Work out the finished part from the listing and answer in its coordinate system (mm). Face numbers are marked on the shaded views. A direction names the side the tool comes from. Coordinates: 2 decimals unless noted, no trailing zeros. Loops run counter-clockwise (first coordinate to the right, second up) from the corner with the lowest first, then second, coordinate; pieces in that order, holes last. Notation, with made-up numbers: (29.5, -33) -> (66.5, -33) arc R22 cw to (66.5, -10) -> close; hole circle Ø7 at (56, 51.5). An arc over 180 degrees is marked (long way). Answer as CSV lines item,"result".
```python
from build123d import *

# Parameters (mm, degrees)
SKETCH2_W               = 60
SKETCH2_H               = 60
BOSS_EXTRUDE1_DEPTH     = 170
SKETCH3_W               = 15
SKETCH3_H               = 60
BOSS_EXTRUDE2_DEPTH     = 30
BOSS_EXTRUDE3_DEPTH     = 15
BOSS_EXTRUDE4_START     = -15
BOSS_EXTRUDE4_DEPTH     = 15
SKETCH6_W               = 60
SKETCH6_H               = 27
BOSS_EXTRUDE5_DEPTH     = 30
BOSS_EXTRUDE6_DEPTH     = 27
CUT_EXTRUDE2_DEPTH      = 5
CUT_EXTRUDE2_DEPTH_BACK = 130
CUT_EXTRUDE2_START      = -10
SKETCH8_W               = 50.5
SKETCH8_H               = 50.5
SKETCH9_R               = 11.35
CUT_EXTRUDE3_DEPTH      = 130
SKETCH11_R              = 3.95
CUT_EXTRUDE4_DEPTH      = 232.543759953
SKETCH12_R              = 3.95
CUT_EXTRUDE5_DEPTH      = 232.543759953
CUT_EXTRUDE7_DEPTH      = 30
FILLET2_R               = 5
FILLET3_R               = 5
SKETCH16_W              = 16
SKETCH16_H              = 11.5
CUT_EXTRUDE8_DEPTH      = 71


with BuildPart() as part:
    # Sketch2 → Boss-Extrude1 (new body)
    with BuildSketch(Plane.XY):
        Rectangle(SKETCH2_W, SKETCH2_H)
    extrude(amount=BOSS_EXTRUDE1_DEPTH)

    # Sketch3 → Boss-Extrude2 (add)
    with BuildSketch(Plane(origin=(0, 0, 0), x_dir=(-1, 0, 0), z_dir=(0, 0, -1))):
        with Locations((22.5, 0)):
            Rectangle(SKETCH3_W, SKETCH3_H)
        with Locations((-22.5, 0)):
            Rectangle(SKETCH3_W, SKETCH3_H)
    extrude(amount=BOSS_EXTRUDE2_DEPTH)

    # Sketch4 → Boss-Extrude3 (add)
    with BuildSketch(Plane(origin=(30, 0, 0), x_dir=(0, 0, -1), z_dir=(1, 0, 0))):
        with BuildLine():
            Line((30, 30), (30, -30))
            ThreePointArc((30, -30), (55.138874415, 0), (30, 30))
        make_face()
    extrude(amount=-BOSS_EXTRUDE3_DEPTH)

    # Sketch5 → Boss-Extrude4 (add)
    with BuildSketch(Plane.ZY.offset(30).offset(BOSS_EXTRUDE4_START)):
        with BuildLine():
            Line((-30, -30), (-30, 30))
            ThreePointArc((-30, 30), (-55.138874415, 0), (-30, -30))
        make_face()
    extrude(amount=BOSS_EXTRUDE4_DEPTH)

    # Sketch6 → Boss-Extrude5 (add)
    with BuildSketch(Plane.XY.offset(170)):
        Rectangle(SKETCH6_W, SKETCH6_H)
    extrude(amount=BOSS_EXTRUDE5_DEPTH)

    # Sketch7 → Boss-Extrude6 (add)
    with BuildSketch(Plane(origin=(0, 13.5, 0), x_dir=(1, 0, 0), z_dir=(0, 1, 0))):
        with BuildLine():
            Line((30, -200), (-30, -200))
            ThreePointArc((-30, -200), (0, -225.138874415), (30, -200))
        make_face()
    extrude(amount=-BOSS_EXTRUDE6_DEPTH)

    # Sketch8 → Cut-Extrude2 (cut, two sides: drawn at the far end of the back side and taken through both)
    with BuildSketch(Plane.XY.offset(170).offset(CUT_EXTRUDE2_START - CUT_EXTRUDE2_DEPTH_BACK)):
        Rectangle(SKETCH8_W, SKETCH8_H)
    extrude(amount=CUT_EXTRUDE2_DEPTH + CUT_EXTRUDE2_DEPTH_BACK, mode=Mode.SUBTRACT)

    # Sketch9 → Cut-Extrude3 (cut)
    with BuildSketch(Plane(origin=(0, -13.5, 0), x_dir=(-1, 0, 0), z_dir=(0, -1, 0))):
        with Locations(Location((0, -200, 0), (0, 0, 90))):
            Circle(SKETCH9_R)
    extrude(amount=-CUT_EXTRUDE3_DEPTH, mode=Mode.SUBTRACT)

    # Sketch11 → Cut-Extrude4 (cut, through all)
    with BuildSketch(Plane.ZY.offset(-15)):
        with Locations(Location((-30, 0, 0), (0, 0, 270))):
            Circle(SKETCH11_R)
    extrude(amount=-CUT_EXTRUDE4_DEPTH, mode=Mode.SUBTRACT)

    # Sketch12 → Cut-Extrude5 (cut, through all)
    with BuildSketch(Plane(origin=(-15, 0, 0), x_dir=(0, 0, -1), z_dir=(1, 0, 0))):
        with Locations(Location((30, 0, 0), (0, 0, 270))):
            Circle(SKETCH12_R)
    extrude(amount=-CUT_EXTRUDE5_DEPTH, mode=Mode.SUBTRACT)

    # Sketch14 → Cut-Extrude7 (cut)
    with BuildSketch(Plane(origin=(-15, 0, 0), x_dir=(0, 0, -1), z_dir=(1, 0, 0))):
        Polygon((0, -30), (0, 0), (-33.188384016, -30), align=None)
        Polygon((-33.188384016, 30), (0, 0), (0, 30), align=None)
    extrude(amount=CUT_EXTRUDE7_DEPTH, mode=Mode.SUBTRACT)

    # Fillet2
    fillet2_edges = [part.edges().sort_by_distance(p)[0] for p in [
        (0, 0, 0),
    ]]
    fillet(fillet2_edges, radius=FILLET2_R)

    # Fillet3
    fillet3_edges = [part.edges().sort_by_distance(p)[0] for p in [
        (0, 13.5, 170),
        (0, -13.5, 170),
    ]]
    fillet(fillet3_edges, radius=FILLET3_R)

    # Sketch16 → Cut-Extrude8 (cut)
    with BuildSketch(Plane(origin=(0, 30, 0), x_dir=(1, 0, 0), z_dir=(0, 1, 0))):
        Polygon((16, -151.43), (16, -101.43), (-16, -101.43), (-16, -139.93), (0, -139.93), (0, -151.43), align=None)
        with Locations((-8, -145.68)):
            Rectangle(SKETCH16_W, SKETCH16_H)
    extrude(amount=-CUT_EXTRUDE8_DEPTH, mode=Mode.SUBTRACT)


solid = part.part
```
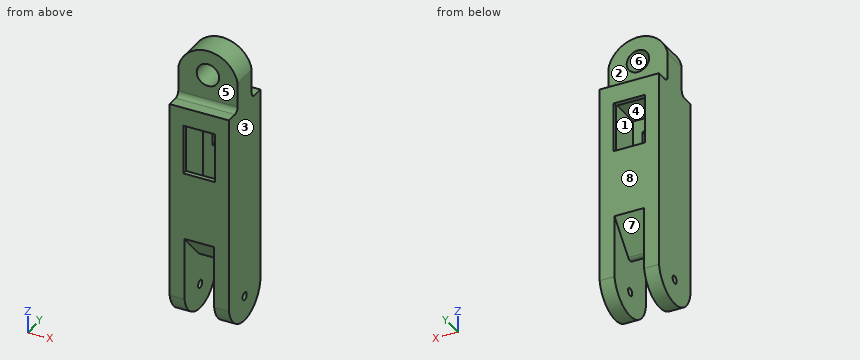
(1) For a pull along X with two mould halves and no side action, classify the marked faces 1, 2 and 3 as pulls with the +X half, pulls with the -X half, needs draft (parallel to the pull), parting line crosses it, or undercut.
Computed values:
face 1,"undercut"
face 2,"needs draft"
face 3,"pulls with the +X half"
(2) A cutting plane is placed at C-C, the plane x = 0. Write down the section's boundary in (y, z).
Computed values:
outline,"(-30, 33.19) -> (-3.71, 4.1) arc R5 ccw to (3.71, 4.1) -> (30, 33.19) -> (30, 101.43) -> (25.25, 101.43) -> (25.25, 30) -> (-25.25, 30) -> (-25.25, 101.43) -> (-30, 101.43) -> close; (-30, 151.43) -> (-25.25, 151.43) -> (-25.25, 165) -> (25.25, 165) -> (25.25, 151.43) -> (30, 151.43) -> (30, 170) -> (18.5, 170) arc R5 cw to (13.5, 175) -> (13.5, 188.65) -> (-13.5, 188.65) -> (-13.5, 175) arc R5 cw to (-18.5, 170) -> (-30, 170) -> close; (-13.5, 211.35) -> (13.5, 211.35) -> (13.5, 225.14) -> (-13.5, 225.14) -> close"
(3) A cutting plane is placed at D-D, the plane y = 21.5. Write down the section's boundary in (x, z) (3 decimals), and give its area (3 significant figures).
Computed values:
outline,"(-30, -46.26) -> (-15, -46.26) -> (-15, 23.785) -> (15, 23.785) -> (15, -46.26) -> (30, -46.26) -> (30, 170) -> (-30, 170) -> close; hole (-25.25, 30) -> (25.25, 30) -> (25.25, 165) -> (-25.25, 165) -> close"
area,"4,060 mm2"
(4) Consider line 1 along X through (y, z) = (7, 200); line 2 along X through (y, z) = (18.5, 131); line 3 along Z through (x, y) = (-20, 0). Determine where each line is inside the solid, lowest interval first.
Computed values:
line 1,"-30 to -11.35, 11.35 to 30"
line 2,"-30 to -25.25, 25.25 to 30"
line 3,"-55.14 to -33.95, -26.05 to 30, 165 to 217.66"
(5) Which of the six approach directions +Z, -Z, +X, -X, +Y, -Y give full straight-line access (tool end or side, diameter ignored) to the marked faces 4, 5, 6, 7 and 8?
Computed values:
face 4,"none"
face 5,"+Z, +X, -X, -Y"
face 6,"+Y, -Y"
face 7,"-Z, +Y"
face 8,"+Z, -Z, +X, -X, +Y"
(6) A cutting plane is placed at A-A, the plane y = 0. Write down the section's boundary in (x, z).
Computed values:
outline,"(-30, -55.14) -> (-15, -55.14) -> (-15, -33.95) -> (-30, -33.95) -> close; (-30, -26.05) -> (-15, -26.05) -> (-15, 2.46) -> (15, 2.46) -> (15, -26.05) -> (30, -26.05) -> (30, 200) arc R30.47 ccw to (-30, 200) -> close; (15, -55.14) -> (30, -55.14) -> (30, -33.95) -> (15, -33.95) -> close; hole (-25.25, 30) -> (25.25, 30) -> (25.25, 165) -> (-25.25, 165) -> close; hole circle Ø22.7 at (0, 200)"
(7) A cutting plane is placed at B-B, the plane z = 137. Write down the section's boundary in (x, y).
Computed values:
outline,"(-30, -30) -> (-16, -30) -> (-16, -25.25) -> (-25.25, -25.25) -> (-25.25, 25.25) -> (-16, 25.25) -> (-16, 30) -> (-30, 30) -> close; (16, -30) -> (30, -30) -> (30, 30) -> (16, 30) -> (16, 25.25) -> (25.25, 25.25) -> (25.25, -25.25) -> (16, -25.25) -> close"
(8) Flat-ended cylindrical pins translate along their axes: pin 1 Ø6 at (x, z) = (23, 192.5) entering from +Y; pin 2 Ø1.5 at (x, y) = (-1, 8.5) entering from +Z; pin 3 Ø5 at (x, z) = (-11, 187) entering from -Y. Find the tip coordinate at first contact, or state that the pin passes through.
Computed values:
pin 1,"y = 13.5"
pin 2,"z = 225.14"
pin 3,"y = -13.5"
